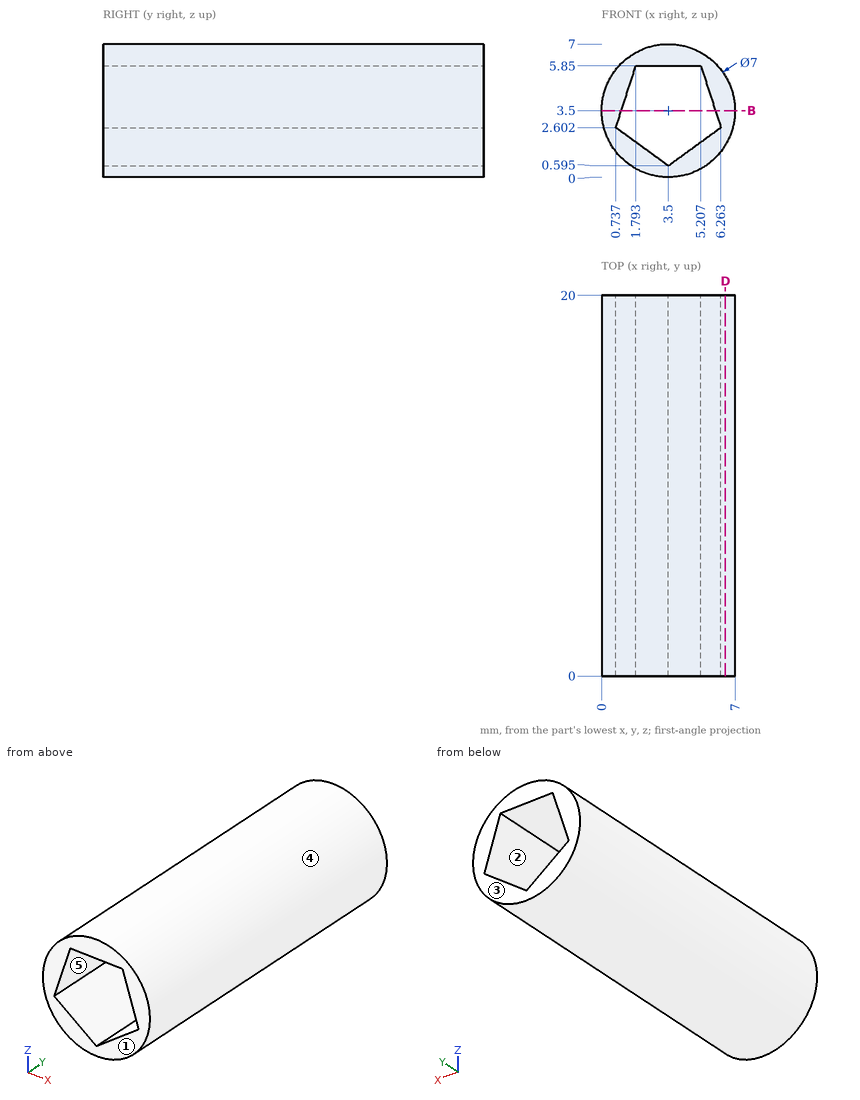
Verification items for this drawing (mm, ordinates from the low corner). A direction names the side the tool comes from. Coordinates: 2 decimals unless noted, no trailing zeros. Loops run counter-clockwise (first coordinate to the right, second up) from the corner with the lowest first, then second, coordinate; pieces in that order, holes last. Notation, with made-up numbers: (81.25, 6.5) -> (126.25, 6.5) arc R15 cw to (126.25, 16.5) -> close; hole circle Ø7 at (61.5, 62). An arc over 180 degrees is marked (long way). Answer in a Markdown table with one row per item. Add a question column.
1. Draft check along Z on the marked faces 3, 4 and 5. Enter one of: +Z half, -Z half, draft (parallel to the pull), parting line (faces both ways), or undercut.
2. Access from +Z, -Z, +X, -X, +Y, -Y to the whole of each face (thin tool, end or side, straight path). Record for the marked faces 1 and 2.
3. Depth check by flat-ended pin: P1, Ø1.5, axis at y = 15.5, z = 1, coming from the +X side; P2, Ø3, axis at x = 4, y = 10.5, coming from the +Z side; P3, Ø1, axis at y = 8, z = 6.5, coming from the +X side; P4, Ø1, axis at x = 5.5, y = 17.5, coming from the -Z side. Enter the tip coordinate at first touch or a pass-through.
4. Material ranges on probe 1 along X at (y, z) = (1, 3.25); probe 2 along X at (y, z) = (15.5, 4) (1 decimal); probe 3 along Z at (x, y) = (0.5, 4.5) (1 decimal), recorded low to high. Write a range as [from, to].
5. Section check D-D, the plane x = 6.5. Enter the section's corners in (y, z), then the cut area to 3 significant figures.
6. Section check B-B, the plane z = 3.5. Enter the section's corners in (x, y).
Derived:
| question | item | result |
|---|---|---|
| 1 | face 3 | draft |
| 1 | face 4 | parting line |
| 1 | face 5 | undercut |
| 2 | face 1 | +Z, -Z, +X, -X, -Y |
| 2 | face 2 | +Y, -Y |
| 3 | P1 | stops at x = 6.53 |
| 3 | P2 | stops at z = 7 |
| 3 | P3 | stops at x = 5.95 |
| 3 | P4 | stops at z = 0.34 |
| 4 | probe 1 | x = [0.01, 0.95], [6.05, 6.99] |
| 4 | probe 2 | x = [0, 1.2], [5.8, 7] |
| 4 | probe 3 | z = [1.7, 5.3] |
| 5 | outline | (0, 1.7) -> (20, 1.7) -> (20, 5.3) -> (0, 5.3) -> close |
| 5 | area | 72.1 mm² |
| 6 | outline | (0, 0) -> (1.03, 0) -> (1.03, 20) -> (0, 20) -> close; (5.97, 0) -> (7, 0) -> (7, 20) -> (5.97, 20) -> close |
